Design review of the part built by this model. Coordinates are the model's own, in mm. Give positions to 0.01 mm unless a question says otherwise; leave off trailing zeros. Order: outer loops, then holes, each group sorted by start corner. A loop starts at its lowest first (then second) coordinate and runs counter-clockwise, first axis right, second up. Notation, with made-up numbers: (-9.5, -11) - (2.5, -11) arc R14 cw to (2.5, -1) - close; hole circle Ø8 at (28.25, 4.25). An arc over 180 degrees is marked (long way). Write each question's results on one line, items separated by ' | '. Start each with the question number.
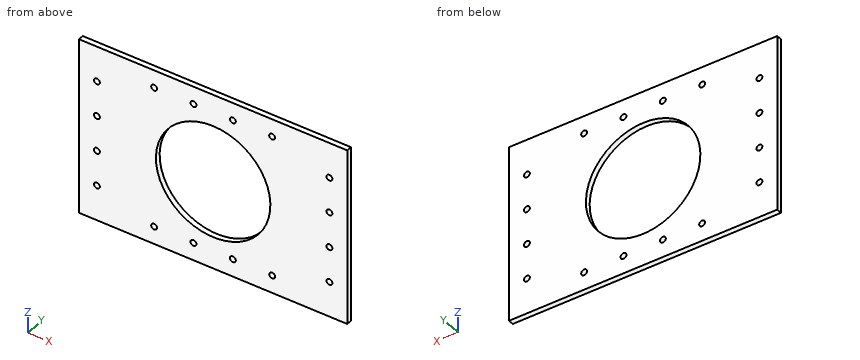
```python
from build123d import *

# Parameters (mm, degrees)
SKETCH_1_W      = 150
SKETCH_1_H      = 100
SKETCH_1_R      = 32
SKETCH_1_R_2    = 1.65
EXTRUDE_1_DEPTH = 3


with BuildPart() as part:
    # 草图1 → 凸台-拉伸1 (new body)
    with BuildSketch(Plane(origin=(0, 0, 0), x_dir=(1, 0, 0), z_dir=(0, 1, 0))):
        Rectangle(SKETCH_1_W, SKETCH_1_H)
        with Locations(Location((0, 0, 0), (0, 0, 270))):
            Circle(SKETCH_1_R, mode=Mode.SUBTRACT)
        with Locations(Location((-65, 30, 0), (0, 0, 270))):
            Circle(SKETCH_1_R_2, mode=Mode.SUBTRACT)
        with Locations(Location((-65, 10, 0), (0, 0, 270))):
            Circle(SKETCH_1_R_2, mode=Mode.SUBTRACT)
        with Locations(Location((-65, -10, 0), (0, 0, 270))):
            Circle(SKETCH_1_R_2, mode=Mode.SUBTRACT)
        with Locations(Location((-65, -30, 0), (0, 0, 270))):
            Circle(SKETCH_1_R_2, mode=Mode.SUBTRACT)
        with Locations(Location((65, -30, 0), (0, 0, 90))):
            Circle(SKETCH_1_R_2, mode=Mode.SUBTRACT)
        with Locations(Location((65, -10, 0), (0, 0, 90))):
            Circle(SKETCH_1_R_2, mode=Mode.SUBTRACT)
        with Locations(Location((65, 10, 0), (0, 0, 90))):
            Circle(SKETCH_1_R_2, mode=Mode.SUBTRACT)
        with Locations(Location((65, 30, 0), (0, 0, 90))):
            Circle(SKETCH_1_R_2, mode=Mode.SUBTRACT)
        with Locations(Location((33, 40, 0), (0, 0, 270))):
            Circle(SKETCH_1_R_2, mode=Mode.SUBTRACT)
        with Locations(Location((11, 40, 0), (0, 0, 270))):
            Circle(SKETCH_1_R_2, mode=Mode.SUBTRACT)
        with Locations(Location((-11, 40, 0), (0, 0, 270))):
            Circle(SKETCH_1_R_2, mode=Mode.SUBTRACT)
        with Locations(Location((-33, 40, 0), (0, 0, 270))):
            Circle(SKETCH_1_R_2, mode=Mode.SUBTRACT)
        with Locations(Location((33, -40, 0), (0, 0, 90))):
            Circle(SKETCH_1_R_2, mode=Mode.SUBTRACT)
        with Locations(Location((11, -40, 0), (0, 0, 90))):
            Circle(SKETCH_1_R_2, mode=Mode.SUBTRACT)
        with Locations(Location((-11, -40, 0), (0, 0, 90))):
            Circle(SKETCH_1_R_2, mode=Mode.SUBTRACT)
        with Locations(Location((-33, -40, 0), (0, 0, 90))):
            Circle(SKETCH_1_R_2, mode=Mode.SUBTRACT)
    extrude(amount=EXTRUDE_1_DEPTH)


solid = part.part
```
Q1. Add section D-D (z = 0). Give the boundary of the cut face in (x, y), plus the area to 3 significant figures.
Q2. Insertion check: pin 1 Ø2.5 at (x, z) = (-33, -40) entering from +Y; pin 2 Ø4 at (x, z) = (65, -10) entering from -Y. Each pin has a flat end and moves straight along its axis. Give the tip position at first contact, or say it passes through.
Q3. For line 1 (Z direction, x = 65, y = 2); line 2 (X direction, y = 0.6, z = 40); line 3 (Z direction, x = 0.5, y = 1.05), list the stretches that pass through material, from the lowest coordinate up. Write a range as [from, to].
Q4. Add section C-C (x = 65). Give the boundary of the cut face in (y, z).
Q5. Add section A-A (z = -40). Give the boundary of the cut face in (x, y), plus the area to 3 significant figures.
Q6. Add section B-B (y = 1.05). Give the number of separate pieces and of enclosed holes in the cut face, plus the area to 3 significant figures.
Verdict:
1) outline: (-75, 0) - (-32, 0) - (-32, 3) - (-75, 3) - close; (32, 0) - (75, 0) - (75, 3) - (32, 3) - close | area: 258 mm2
2) pin 1: passes through | pin 2: stops at y = 0
3) line 1: z = [-50, -31.65], [-28.35, -11.65], [-8.35, 8.35], [11.65, 28.35], [31.65, 50] | line 2: x = [-75, -34.65], [-31.35, -12.65], [-9.35, 9.35], [12.65, 31.35], [34.65, 75] | line 3: z = [-50, -32], [32, 50]
4) outline: (0, -50) - (3, -50) - (3, -31.65) - (0, -31.65) - close; (0, -28.35) - (3, -28.35) - (3, -11.65) - (0, -11.65) - close; (0, -8.35) - (3, -8.35) - (3, 8.35) - (0, 8.35) - close; (0, 11.65) - (3, 11.65) - (3, 28.35) - (0, 28.35) - close; (0, 31.65) - (3, 31.65) - (3, 50) - (0, 50) - close
5) outline: (-75, 0) - (-34.65, 0) - (-34.65, 3) - (-75, 3) - close; (-31.35, 0) - (-12.65, 0) - (-12.65, 3) - (-31.35, 3) - close; (-9.35, 0) - (9.35, 0) - (9.35, 3) - (-9.35, 3) - close; (12.65, 0) - (31.35, 0) - (31.35, 3) - (12.65, 3) - close; (34.65, 0) - (75, 0) - (75, 3) - (34.65, 3) - close | area: 410 mm2
6) separate pieces: 1 | enclosed holes: 17 | area: 11,600 mm2
